Part model, mm, in its own coordinate system. Give positions to 0.01 mm unless a question says otherwise; leave off trailing zeros. Order: outer loops, then holes, each group sorted by start corner. A loop starts at its lowest first (then second) coordinate and runs counter-clockwise, first axis right, second up. Notation, with made-up numbers: M -22.75,2 L 26.25,2 A27 cw 26.25,21 Z; hole C -22,1 d6. An arc over 180 degrees is marked long. One line per question, with ' | ' between items.
```python
from build123d import *

# Parameters (mm, degrees)
F0_W     = 30
F0_H     = 20
F1_DEPTH = 10
F3_D     = 1.54


with BuildPart() as f1:
    # F0 (on Front) → F1 (new body, symmetric)
    with BuildSketch(Plane.XZ):
        Rectangle(F0_W, F0_H)
    extrude(amount=F1_DEPTH, both=True)

    # F3 (through all)
    with Locations(Plane.XZ.offset(10)):
        with Locations((-10, 0), (0, 0), (10, 0)):
            Hole(F3_D / 2)


solid = f1.part
```
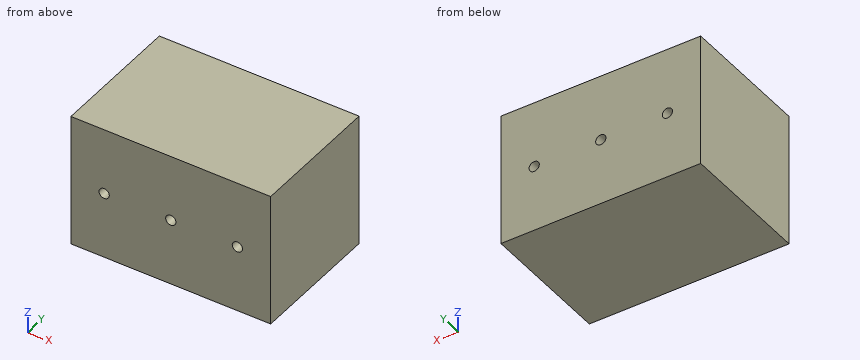
1. Slice it at B-B on x = 10. Give the cut face in (y, z).
Worked out:
outline: M -10,-10 L 10,-10 L 10,-0.77 L -10,-0.77 Z; M -10,0.77 L 10,0.77 L 10,10 L -10,10 Z
2. Slice it at A-A on z = 0. Give the cut face in (x, y), then the cut area to 3 significant figures.
Worked out:
outline: M -15,-10 L -10.77,-10 L -10.77,10 L -15,10 Z; M -9.23,-10 L -0.77,-10 L -0.77,10 L -9.23,10 Z; M 0.77,-10 L 9.23,-10 L 9.23,10 L 0.77,10 Z; M 10.77,-10 L 15,-10 L 15,10 L 10.77,10 Z | area: 508 mm2
3. Probe L1, parallel to Z at x = 10, y = -2.25; L2, parallel to X at y = -2.5, z = 0.5; L3, parallel to X at y = 4, z = 0.25. List the from-to ranges inside material, lowest first. Write a range as from..to.
Worked out:
L1: z = -10..-0.77, 0.77..10 | L2: x = -15..-10.59, -9.41..-0.59, 0.59..9.41, 10.59..15 | L3: x = -15..-10.73, -9.27..-0.73, 0.73..9.27, 10.73..15
